Autodesk Inventor part; units mm, degrees
ref_plane "YZ Plane" through (0, 0, 0) normal (1, 0, 0) x (0, 1, 0)
ref_plane "XZ Plane" through (0, 0, 0) normal (0, 1, 0) x (-1, 0, 0)
ref_plane "XY Plane" through (0, 0, 0) normal (0, 0, 1) x (1, 0, 0)
sketch "Эскиз1" plane through (0, 0, 0) normal (0, 0, 1) x (1, 0, 0)
  line L0 (0, 0) -> (-54.5, 0)
  line L1 (-54.5, 0) -> (-54.5, -15)
  line L2 (-54.5, -15) -> (-50.5, -15)
  line L3 (-50.5, -15) -> (-50.5, -30)
  line L4 (-50.5, -30) -> (-40.5, -30)
  line L5 (-40.5, -30) -> (-40.5, -34)
  line L6 (-40.5, -34) -> (-11.5, -34)
  line L7 (-11.5, -34) -> (-11.5, -30)
  line L8 (-54.5, 0) -> (-54.5, 15)
  line L9 (-54.5, 15) -> (-50.5, 15)
  line L10 (-50.5, 15) -> (-50.5, 30)
  line L11 (-50.5, 30) -> (-40.5, 30)
  line L12 (-40.5, 30) -> (-40.5, 34)
  line L13 (-40.5, 34) -> (-11.5, 34)
  line L14 (-11.5, 34) -> (-11.5, 30)
  line L15 (-11.5, -30) -> (-4, -30)
  line L16 (-4, -30) -> (-4, -15)
  line L17 (-4, -15) -> (0, -15)
  line L18 (0, -15) -> (0, 0)
  line L19 (-11.5, 30) -> (-4, 30)
  line L20 (-4, 30) -> (-4, 15)
  line L21 (-4, 15) -> (0, 15)
  line L22 (0, 15) -> (0, 0)
  dimension "d0" = 29
  dimension "d2" = 10
  dimension "d3" = 30
  dimension "d4" = 15
  dimension "d5" = 4
  dimension "d8" = 11.5
  dimension "d9" = 4
extrude "Выдавливание1" add sketch "Эскиз1" along normal blind 4
properties part number "topRL"
Geometry check sheet. Reference: the model listing, model coordinates, mm. A direction names the side the tool comes from. Give positions to 0.01 mm unless a question says otherwise; leave off trailing zeros. Order: outer loops, then holes, each group sorted by start corner. A loop starts at its lowest first (then second) coordinate and runs counter-clockwise, first axis right, second up. Notation, with made-up numbers: (84.25, -6.5) - (99.25, -6.5) arc R27 ccw to (99.25, 24.5) - close; hole circle Ø11 at (-15, -13). An arc over 180 degrees is marked (long way). Answer in a Markdown table with one row per item. Add a question column.
Q1. Cross-section at C-C, the plane y = 16.5. Enter the section's corners in (x, z), then the cut area to 3 significant figures.
Q2. Tool access check on faces 1 (the flat face through (-40.5, 32, 2)), 2 (the flat face through (-4, 23, 2)), 3 (the flat face through (-2, -15, 2)), 4 (the flat face through (-46, -30, 2)). Record the directions out of +Z, -Z, +X, -X, +Y, -Y that give a thin tool (end or side, any length) a straight path to the whole face; none if there is none.
Q3. Gauge pin test, flat ends, axial feed: pin 1 (1.2 mm diameter, centred on x = -52, z = 1, fed in from +Y); pin 2 (2 mm diameter, centred on y = -20, z = 2.5, fed in from +X); pin 3 (1.5 mm diameter, centred on x = -10, z = 3, fed in from -Y). Record the tip position at first contact, or that the pin passes through.
Q4. Cross-section at B-B, the plane x = -6. Enter the section's corners in (y, z).
Q5. Material ranges on probe 1 along X at (y, z) = (26, 0.2); probe 2 along X at (y, z) = (-31, 3.1); probe 3 along Y at (x, z) = (-49, 0.4), recorded low to high. Write a range as from..to.
Q6. Cross-section at A-A, the plane z = 1.5. Enter the section's corners in (x, y).
Check values:
| question | item | result |
|---|---|---|
| 1 | outline | (-50.5, 0) - (-4, 0) - (-4, 4) - (-50.5, 4) - close |
| 1 | area | 186 mm^2 |
| 2 | face 1 | +Z, -Z, -X, +Y |
| 2 | face 2 | +Z, -Z, +X, +Y |
| 2 | face 3 | +Z, -Z, +X, -Y |
| 2 | face 4 | +Z, -Z, -X, -Y |
| 3 | pin 1 | stops at y = 15 |
| 3 | pin 2 | stops at x = -4 |
| 3 | pin 3 | stops at y = -30 |
| 4 | outline | (-30, 0) - (30, 0) - (30, 4) - (-30, 4) - close |
| 5 | probe 1 | x = -50.5..-4 |
| 5 | probe 2 | x = -40.5..-11.5 |
| 5 | probe 3 | y = -30..30 |
| 6 | outline | (-54.5, -15) - (-50.5, -15) - (-50.5, -30) - (-40.5, -30) - (-40.5, -34) - (-11.5, -34) - (-11.5, -30) - (-4, -30) - (-4, -15) - (0, -15) - (0, 15) - (-4, 15) - (-4, 30) - (-11.5, 30) - (-11.5, 34) - (-40.5, 34) - (-40.5, 30) - (-50.5, 30) - (-50.5, 15) - (-54.5, 15) - close |
